Verification items for the finished model (mm, model axes). A direction names the side the tool comes from. Give positions to 0.01 mm unless a question says otherwise; leave off trailing zeros. Order: outer loops, then holes, each group sorted by start corner. A loop starts at its lowest first (then second) coordinate and runs counter-clockwise, first axis right, second up. Notation, with made-up numbers: (14, 7) -> (27, 7) arc R9 ccw to (27, 17) -> close; hole circle Ø6 at (16.25, 26). An arc over 180 degrees is marked (long way). Return JSON: item names as keys, results as strings. Group by question number.
(1) Release check for a two-part mould opening along Z. For faces 4 (the face through (6, 0, 50)), 5 (the face through (0, 28.015, 1)) record: pulls with the +Z half, pulls with the -Z half, needs draft (parallel to the pull), parting line crosses it, or undercut.
(2) Thickness scan on line 1 along X through (y, z) = (8, -11.5); line 2 along Z through (x, y) = (-23, 1); line 3 along Y through (x, z) = (-7, 6). Record the ranges inside material, lowest first.
(3) Depth check by flat-ended pin: pin 1 Ø2 at (x, y) = (-16.5, 22.5) entering from -Z; pin 2 Ø10 at (x, y) = (-32, 7) entering from -Z; pin 3 Ø16.5 at (x, y) = (9, 12.5) entering from +Z; pin 4 Ø10 at (y, z) = (-34, -34.5) entering from -X. Enter the tip coordinate at first touch or a pass-through.
(4) Cross-section at B-B on y = -30.5. Enter the section's corners in (x, z), then the cut area to 3 significant figures.
(5) Cross-section at C-C on x = -33. Enter the section's corners in (y, z).
(6) Cross-section at A-A on z = 16.5. Enter the section's corners in (x, y).
(7) Tool access check on faces 1 (the face through (27.91, 0, 1)), 2 (the face through (-27.91, 0, 1)), 3 (the face through (0, -28.015, 1)). Record the directions out of +Z, -Z, +X, -X, +Y, -Y that give a thin tool (end or side, any length) a straight path to the whole face; none if there is none.
from build123d import *

# Parameters (mm, degrees)
F0_W      = 55.819296
F0_H      = 56.029066
F1_DEPTH  = 50
F1_FACE_W = 55.819296
F1_FACE_H = 56.029066
F5_R      = 0.01


with BuildPart() as f1:
    # F0 (on Top) → F1 (new body, symmetric)
    with BuildSketch(Plane.XY):
        Rectangle(F0_W, F0_H)
    extrude(amount=F1_DEPTH, both=True)

    # F2 (on Right) → F3 (revolve)
    with BuildSketch(Plane.YZ):
        with BuildLine():
            Line((0, 49.893861), (0, 148.123125))
            ThreePointArc((0, 148.123125), (-49.114632, 99.008493), (0, 49.893861))
        make_face()
    revolve(axis=Axis((0, 0, 99.008493), (0, 0, 1)))

    # F1_face (on face) → F6 section 0
    with BuildSketch(Plane(origin=(0, 0, -50), x_dir=(1, 0, 0), z_dir=(0, 0, -1))):
        Rectangle(F1_FACE_W, F1_FACE_H)
    # F5 (on offset) → F6 section 1
    with BuildSketch(Plane.XY.offset(-75)):
        Circle(F5_R)
    loft()


solid = f1.part
Verdict:
{
 "1": {"face 4": "undercut", "face 5": "needs draft"},
 "2": {"line 1": "-27.91 to 27.91", "line 2": "-54.4 to 50, 55.62 to 142.39", "line 3": "-28.01 to 28.01"},
 "3": {"pin 1": "z = -55.82", "pin 2": "z = -50.82", "pin 3": "z = 147.6", "pin 4": "through"},
 "4": {"outline": "circle Ø76.99 at (0, 99.01)", "area": "4,660 mm²"},
 "5": {"outline": "circle Ø72.75 at (0, 99.01)"},
 "6": {"outline": "(-27.91, -28.01) -> (27.91, -28.01) -> (27.91, 28.01) -> (-27.91, 28.01) -> close"},
 "7": {"face 1": "-Z, +X, +Y, -Y", "face 2": "-Z, -X, +Y, -Y", "face 3": "-Z, +X, -X, -Y"}
}
